Verification items for the finished model (mm, model axes). A direction names the side the tool comes from. Coordinates: 2 decimals unless noted, no trailing zeros. Loops run counter-clockwise (first coordinate to the right, second up) from the corner with the lowest first, then second, coordinate; pieces in that order, holes last. Notation, with made-up numbers: (38, 74.25) -> (59, 74.25) arc R16 ccw to (59, 90.25) -> close; hole circle Ø3 at (60.25, 36). An arc over 180 degrees is marked (long way). Write item = value, one per line.
```python
from build123d import *

# Parameters (mm, degrees)
SKETCH1_R           = 30
BOSS_EXTRUDE2_DEPTH = 25
SKETCH1_3_R         = 10
BOSS_EXTRUDE3_DEPTH = 20
CUT_EXTRUDE2_DEPTH  = 112.467484048


with BuildPart() as part:
    # Sketch1 → Boss-Extrude2 (new, symmetric)
    with BuildSketch(Plane.YZ):
        with Locations(Location((0, 0, 0), (0, 0, 270))):
            Circle(SKETCH1_R)
    extrude(amount=BOSS_EXTRUDE2_DEPTH, both=True)

    # Sketch1_3 → Boss-Extrude3 (add)
    with BuildSketch(Plane.YZ):
        with BuildLine():
            ThreePointArc((75, -20), (95, 0), (75, 20))
            Line((75, 20), (22.360679775, 20))
            ThreePointArc((22.360679775, 20), (28.025170769, 10.704662693), (30, 0))
            ThreePointArc((30, 0), (28.025170769, -10.704662693), (22.360679775, -20))
            Line((22.360679775, -20), (75, -20))
        make_face()
        with Locations(Location((75, 0, 0), (0, 0, 270))):
            Circle(SKETCH1_3_R, mode=Mode.SUBTRACT)
    extrude(amount=-BOSS_EXTRUDE3_DEPTH)

    # Sketch3 → Cut-Extrude2 (cut, through all)
    with BuildSketch(Plane.YZ.offset(25)):
        with BuildLine():
            Line((-4, 20.522711642), (4, 20.522711642))
            Line((4, 20.522711642), (4, 16.522711642))
            ThreePointArc((4, 16.522711642), (0, -17), (-4, 16.522711642))
            Line((-4, 16.522711642), (-4, 20.522711642))
        make_face()
    extrude(amount=-CUT_EXTRUDE2_DEPTH, mode=Mode.SUBTRACT)


solid = part.part
```
1) Tool access check on faces 1 (the face through (-10, 48, -20)), 2 (the face through (0, 4, 19)), 3 (the face through (-10, 49, 20)). Record the directions out of +Z, -Z, +X, -X, +Y, -Y that give a thin tool (end or side, any length) a straight path to the whole face; none if there is none.
Ans:
face_1 = -Z, +X, -X, +Y
face_2 = +X, -X
face_3 = +Z, +X, -X, +Y
2) Sectioned sample at A-A, the plane y = 0. Record the cut outline in (x, z).
Ans:
outline = (-25, -30) -> (25, -30) -> (25, -17) -> (-25, -17) -> close; (-25, 20.52) -> (25, 20.52) -> (25, 30) -> (-25, 30) -> close
3) Material ranges on line 1 (Y direction, x = -14, z = 0); line 2 (Y direction, x = -10.5, z = -5); line 3 (Z direction, x = -6.5, y = 39.5), recorded low to high.
Ans:
line_1 = -30 to -17, 17 to 65, 85 to 95
line_2 = -29.58 to -16.25, 16.25 to 66.34, 83.66 to 94.36
line_3 = -20 to 20
4) Sectioned sample at D-D, the plane x = 4.5. Record the cut outline in (y, z).
Ans:
outline = circle Ø60 at (0, 0); hole (-4, 16.52) arc R17 ccw (long way) to (4, 16.52) -> (4, 20.52) -> (-4, 20.52) -> close
5) Sectioned sample at C-C, the plane x = -6. Record the cut outline in (y, z), plus the area to 3 significant figures.
Ans:
outline = (22.36, -20) -> (75, -20) arc R20 ccw to (75, 20) -> (22.36, 20) arc R30 ccw (long way) to start; hole (-4, 16.52) arc R17 ccw (long way) to (4, 16.52) -> (4, 20.52) -> (-4, 20.52) -> close; hole circle Ø20 at (75, 0)
area = 4,100 mm2
6) Depth check by flat-ended pin: pin 1 Ø5 at (y, z) = (65.5, -19.5) entering from +X; pin 2 Ø12 at (x, y) = (-6.5, 49.5) entering from +Z; pin 3 Ø1 at (y, z) = (23.5, 21.5) entering from -X; pin 4 Ø5 at (y, z) = (25.5, 18) entering from +X. Enter the tip coordinate at first touch or a pass-through.
Ans:
pin_1 = 0
pin_2 = 20
pin_3 = through
pin_4 = 25
7) Sectioned sample at B-B, the plane z = 0. Record the cut outline in (x, y).
Ans:
outline = (-25, -30) -> (25, -30) -> (25, -17) -> (-25, -17) -> close; (-25, 17) -> (25, 17) -> (25, 30) -> (0, 30) -> (0, 65) -> (-20, 65) -> (-20, 30) -> (-25, 30) -> close; (-20, 85) -> (0, 85) -> (0, 95) -> (-20, 95) -> close
